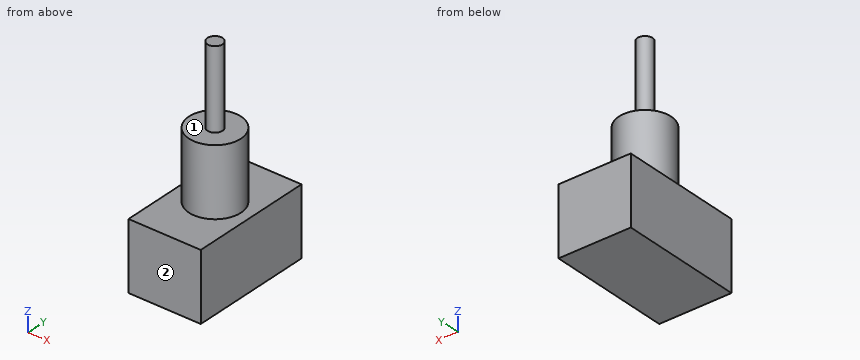
```python
from build123d import *

# Parameters (mm, degrees)
F0_R     = 5.842
F1_DEPTH = 15.24
F2_R     = 1.696679
F3_DEPTH = 17.78
F4_W     = 16.256
F4_H     = 27.940002
F5_DEPTH = 15.24


with BuildPart() as f1:
    # F0 (on Top) → F1 (new body)
    with BuildSketch(Plane.XY):
        Circle(F0_R)
    extrude(amount=F1_DEPTH)

    # F2 (on face) → F3 (join)
    with BuildSketch(Plane.XY.offset(15.24)):
        Circle(F2_R)
    extrude(amount=F3_DEPTH)

    # F4 (on Top) → F5 (join)
    with BuildSketch(Plane.XY):
        Rectangle(F4_W, F4_H)
    extrude(amount=-F5_DEPTH)


solid = f1.part
```
CAD build for the part. Positions are in the model's coordinates, mm. Face numbers are marked on the shaded views. A direction names the side the tool comes from. Coordinates: 2 decimals unless noted, no trailing zeros. Order: outer loops, then holes, each group sorted by start corner. A loop starts at its lowest first (then second) coordinate and runs counter-clockwise, first axis right, second up.
(1) Drill centre lines: L1, parallel to Z at x = 0.25, y = 8; L2, parallel to Z at x = -0.75, y = -3; L3, parallel to Y at x = 0, z = 1.5. Where is each one in solid material? Low to high.
Solution:
L1: z = -15.24 to 0
L2: z = -15.24 to 15.24
L3: y = -5.84 to 5.84
(2) Saw through at C-C, the plane z = 3.5. Write the cut outline in (x, y).
Solution:
outline: circle Ø11.68 at (0, 0)
(3) Saw through at A-A, the plane y = 0. Write the cut outline in (x, z), and give its area (3 significant figures).
Solution:
outline: (-8.13, -15.24) - (8.13, -15.24) - (8.13, 0) - (5.84, 0) - (5.84, 15.24) - (1.7, 15.24) - (1.7, 33.02) - (-1.7, 33.02) - (-1.7, 15.24) - (-5.84, 15.24) - (-5.84, 0) - (-8.13, 0) - close
area: 486 mm2
(4) Which spindle directions (+Z, -Z, +X, -X, +Y, -Y) get a long thin tool onto all of the face, cutting with end or side? Do the marked faces 1 and 2. Say none if no direction does.
Solution:
face 1: +Z
face 2: +Z, -Z, +X, -X, -Y
(5) Saw through at D-D, the plane x = 0. Write the cut outline in (y, z), and give its area (3 significant figures).
Solution:
outline: (-13.97, -15.24) - (13.97, -15.24) - (13.97, 0) - (5.84, 0) - (5.84, 15.24) - (1.7, 15.24) - (1.7, 33.02) - (-1.7, 33.02) - (-1.7, 15.24) - (-5.84, 15.24) - (-5.84, 0) - (-13.97, 0) - close
area: 664 mm2
(6) Pin check, flat tips, straight feed: pin 1 Ø3 at (x, z) = (6, 11) entering from -Y; pin 2 Ø5 at (y, z) = (-7.5, 10) entering from +X; pin 3 Ø3 at (x, y) = (-1, -7) entering from +Z. Stop position of each tip, or through.
Solution:
pin 1: stops at y = -3.73
pin 2: stops at x = 3.02
pin 3: stops at z = 15.24
(7) Saw through at B-B, the plane x = -3.25. Write the cut outline in (y, z).
Solution:
outline: (-13.97, -15.24) - (13.97, -15.24) - (13.97, 0) - (4.85, 0) - (4.85, 15.24) - (-4.85, 15.24) - (-4.85, 0) - (-13.97, 0) - close
